from build123d import *

# Parameters (mm, degrees)
F0_W     = 34.47
F0_H     = 19.95
F1_DEPTH = 5
F2_W     = 24.49
F2_H     = 2.5
F3_DEPTH = 5
F5_DEPTH = 5
F7_DEPTH = 5


with BuildPart() as f1:
    # F0 (on Front) → F1 (new body)
    with BuildSketch(Plane.XZ):
        Rectangle(F0_W, F0_H)
    extrude(amount=-F1_DEPTH)

    # F2 (on face) → F3 (cut, through all)
    with BuildSketch(Plane.XZ):
        with Locations((-4.99, 8.725)):
            Rectangle(F2_W, F2_H)
    extrude(amount=-F3_DEPTH, mode=Mode.SUBTRACT)

    # F4 (on face) → F5 (cut, through all)
    with BuildSketch(Plane.XZ):
        with BuildLine():
            ThreePointArc((-3.265, -5.975), (-2.679214, -7.389214), (-1.265, -7.975))
            Line((-1.265, -7.975), (-1.265, -5.975))
            Line((-1.265, -5.975), (-3.265, -5.975))
        make_face()
        with BuildLine():
            ThreePointArc((-12.265, 1.025), (-13.972107, 1.732107), (-13.265, 0.025))
            ThreePointArc((-13.265, 0.025), (-12.557893, 0.317893), (-12.265, 1.025))
        make_face()
        with BuildLine():
            ThreePointArc((-13.265, -3.975), (-14.679214, -7.389214), (-11.265, -5.975))
            Line((-11.265, -5.975), (-13.265, -5.975))
            Line((-13.265, -5.975), (-13.265, -3.975))
        make_face()
        with BuildLine():
            Line((-13.265, -5.975), (-11.265, -5.975))
            ThreePointArc((-11.265, -5.975), (-11.850786, -4.560786), (-13.265, -3.975))
            Line((-13.265, -3.975), (-13.265, -5.975))
        make_face()
        with BuildLine():
            ThreePointArc((-0.265, 1.025), (-1.972107, 1.732107), (-1.265, 0.025))
            ThreePointArc((-1.265, 0.025), (-0.557893, 0.317893), (-0.265, 1.025))
        make_face()
        with BuildLine():
            Line((-1.265, -5.975), (-1.265, -7.975))
            ThreePointArc((-1.265, -7.975), (0.149214, -7.389214), (0.735, -5.975))
            ThreePointArc((0.735, -5.975), (0.149214, -4.560786), (-1.265, -3.975))
            Line((-1.265, -3.975), (-1.265, -5.975))
        make_face()
        with BuildLine():
            Line((-3.265, -5.975), (-1.265, -5.975))
            Line((-1.265, -5.975), (-1.265, -3.975))
            ThreePointArc((-1.265, -3.975), (-2.679214, -4.560786), (-3.265, -5.975))
        make_face()
    extrude(amount=-F5_DEPTH, mode=Mode.SUBTRACT)

    # F6 (on face) → F7 (cut, through all)
    with BuildSketch(Plane.XZ):
        with BuildLine():
            ThreePointArc((8.235, -4.975), (6.608983, -6.469697), (8.235, -7.964394))
            Line((8.235, -7.964394), (8.235, -4.975))
        make_face()
        with BuildLine():
            Line((8.235, -4.975), (8.235, -7.964394))
            ThreePointArc((8.235, -7.964394), (15.507417, -0.969697), (8.235, 6.025))
            ThreePointArc((8.235, 6.025), (6.735, 4.525), (8.235, 3.025))
            ThreePointArc((8.235, 3.025), (11.063427, 1.853427), (12.235, -0.975))
            ThreePointArc((12.235, -0.975), (11.063427, -3.803427), (8.235, -4.975))
        make_face()
        with BuildLine():
            ThreePointArc((9.735, -0.975), (7.17434, 0.08566), (8.235, -2.475))
            ThreePointArc((8.235, -2.475), (9.29566, -2.03566), (9.735, -0.975))
        make_face()
    extrude(amount=-F7_DEPTH, mode=Mode.SUBTRACT)


solid = f1.part
Could you check a few things on this model? Use its own coordinates, in mm. A direction names the side the tool comes from. Give positions to 0.01 mm unless a question says otherwise; leave off trailing zeros. Loops run counter-clockwise (first coordinate to the right, second up) from the corner with the lowest first, then second, coordinate; pieces in that order, holes last. Notation, with made-up numbers: M 11,-1 L 27,-1 A24 cw 27,38 Z; hole C -14,17.5 d4. An arc over 180 degrees is marked long. Answer as a JSON object with one key per item and string values.
Q1. Suppose I cut it at C-C, the plane y = 1.3. List the corners of the cut face in (x, z) for me (3 decimals).
Values found:
{"outline": "M -17.235,-9.975 L 17.235,-9.975 L 17.235,9.975 L 7.255,9.975 L 7.255,7.475 L -17.235,7.475 Z; hole C -13.265,1.025 d2; hole M -13.265,-3.975 A2 ccw long -11.265,-5.975 A2 ccw Z; hole M -3.265,-5.975 A2 ccw -1.265,-7.975 A2 ccw 0.735,-5.975 A2 ccw -1.265,-3.975 A2 ccw Z; hole C -1.265,1.025 d2; hole C 8.235,-0.975 d3; hole M 8.235,-7.964 A7 ccw long 8.235,6.025 A1.5 ccw 8.235,3.025 A4 cw 8.235,-4.975 A1.5 ccw long Z"}
Q2. Suppose I cut it at B-B, the plane z = 4.5. List the corners of the cut face in (x, y) for me (3 decimals).
Values found:
{"outline": "M -17.235,0 L 6.735,0 L 6.735,5 L -17.235,5 Z; M 12.876,0 L 17.235,0 L 17.235,5 L 12.876,5 Z"}
Q3. If we mould it in two halves opening along X, with no side actions, what happens to faces 4 (the cylindrical face through (6.61, 2.46, -6.43)), 5 (the flat face through (0, 0, 0)), 6 (the flat face through (17.235, 2, 0))? For each: pulls with the +X half, pulls with the -X half, needs draft (parallel to the pull), parting line crosses it, or undercut.
Values found:
{"face 4": "undercut", "face 5": "needs draft", "face 6": "pulls with the +X half"}
Q4. For faces 1 (the flat face through (7.255, 2, 9)), 2 (the flat face through (0, 5, 0)), 3 (the cylindrical face through (15.506, 2.465, -1.127)), which set-ups out of +Z, -Z, +X, -X, +Y, -Y let a thin tool reach every point of the face, with its end or its side?
Values found:
{"face 1": "+Z, -X, +Y, -Y", "face 2": "+Z, -Z, +X, -X, +Y", "face 3": "+Y, -Y"}
Q5. If I drill on probe 1 along X at (y, z) = (1.8, -0.5) (3 decimals); probe 2 along X at (y, z) = (1.3, -2) (3 decimals); probe 3 along Z at (x, y) = (10, 0.5) (3 decimals), over which ranges is the centre line in solid material (lowest first)? Write a range as [from, to].
Values found:
{"probe 1": "x = [-17.235, 6.812], [9.658, 12.207], [15.492, 17.235]", "probe 2": "x = [-17.235, 7.14], [9.33, 12.101], [15.431, 17.235]", "probe 3": "z = [-9.975, -7.809], [-4.565, 2.615], [5.869, 9.975]"}
Q6. Suppose I cut it at D-D, the plane x = 5. List the corners of the cut face in (y, z) for me (3 decimals), plus the area to 4 significant figures.
Values found:
{"outline": "M 0,-9.975 L 5,-9.975 L 5,7.475 L 0,7.475 Z", "area": "87.25 mm²"}
Q7. For P1, Ø1.5, axis at x = -2.5, z = -5.5, coming from the +Y side, with a flat end and sliding along its axis, tell me the tip position at first contact or that it passes through.
Values found:
{"P1": "stops at y = 5"}
Q8. Suppose I cut it at A-A, the plane x = 10.5. List the corners of the cut face in (y, z) for me (3 decimals).
Values found:
{"outline": "M 0,-9.975 L 5,-9.975 L 5,-7.68 L 0,-7.68 Z; M 0,-4.272 L 5,-4.272 L 5,2.322 L 0,2.322 Z; M 0,5.741 L 5,5.741 L 5,9.975 L 0,9.975 Z"}
